Autodesk Inventor part; units mm, degrees
ref_plane "YZ Plane" through (0, 0, 0) normal (1, 0, 0) x (0, 1, 0)
ref_plane "XZ Plane" through (0, 0, 0) normal (0, 1, 0) x (-1, 0, 0)
ref_plane "XY Plane" through (0, 0, 0) normal (0, 0, 1) x (1, 0, 0)
sketch "Sketch1" plane through (0, 0, 0) normal (0, 0, 1) x (1, 0, 0)
  circle A0 centre (0, 0) radius 3.302
  line L0 (0, 0) -> (0, 9.525)
  circle A1 centre (0, 9.525) radius 1.5875
  circle A2 centre (-8.2489, -4.7625) radius 1.5875
  circle A3 centre (8.2489, -4.7625) radius 1.5875
  circle A4 centre (0, 0) radius 12.7
  dimension "d0" = 6.604
  dimension "d1" = 9.525
  dimension "d2" = 3.175
  dimension "d5" = 360
  dimension "d7" = 25.4
extrude "Extrusion1" add sketch "Sketch1" along normal blind 3.175
sketch "Sketch2" plane through (0, 0, 3.175) normal (0, 0, 1) x (1, 0, 0)
  circle A0 centre (0, 0) radius 3.302
  circle A1 centre (8.2489, -4.7625) radius 1.5875
  circle A2 centre (-8.2489, -4.7625) radius 1.5875
  circle A3 centre (0, 9.525) radius 1.5875
  circle A4 centre (0, 0) radius 12.7
  circle A5 centre (0, 0) radius 2.3813
  dimension "d10" = 4.7625
extrude "Extrusion2" add sketch "Sketch2" along normal blind 0.635 contours A0 | A4
chamfer "Chamfer1" distance 1.27 angle 45 3 edges at (-1.5875, 9.525, 0) (-9.8364, -4.7625, 0) (6.6614, -4.7625, 0)
sketch "Sketch3" plane through (0, 0, 0) normal (0, 0, -1) x (-1, 0, 0)
  line L0 (0, 0) -> (17.5976, 10.16)
  line L1 (0, 0) -> (20.32, 0) construction
  circle A0 centre (17.5976, 10.16) radius 11.1125
  circle A1 centre (-17.5976, 10.16) radius 11.1125
  circle A2 centre (0, -20.32) radius 11.1125
  dimension "d16" = 20.32
  dimension "d17" = 30
  dimension "d18" = 22.225
  dimension "d21" = 360
extrude "Extrusion3" cut sketch "Sketch3" against normal blind 25.4
fillet "Fillet1" radius 3.175 6 edges at (-12.6986, 0.1857, 1.905) (-6.5101, 10.9045, 1.905) (12.6986, 0.1857, 1.905) (6.5101, 10.9045, 1.905) (6.1885, -11.0902, 1.905) (-6.1885, -11.0902, 1.905)
properties part number "spoolPinionBearingHolder" material "ABS Plastic"
Source: CAD feature listing. Evaluate the final solid. Frame: model axes, mm. A direction names the side the tool comes from. Round coordinates to 2 decimals unless told otherwise and drop trailing zeros. Order: outer loops, then holes, each group sorted by start corner. A loop starts at its lowest first (then second) coordinate and runs counter-clockwise, first axis right, second up. Notation, with made-up numbers: (27.5, 46.25) -> (54.5, 46.25) arc R25 ccw to (54.5, 59.25) -> close; hole circle Ø8 at (71, 66.25). An arc over 180 degrees is marked (long way). One line per item, written item: value. Start each with the question number.
Q1. Pin query (flat end, axial travel): pin 1 (2 mm diameter, centred on y = -8, z = 2.5, fed in from +X); pin 2 (10 mm diameter, centred on x = -5, y = 3.5, fed in from -Z); pin 3 (5 mm diameter, centred on x = -8.25, y = -4.76, fed in from -Z). Return the tip coordinate at first contact, or that it passes through.
Q2. Access query for faces 5 (the cylindrical face through (3.05, 1.26, 1.57)), 6 (the flat face through (3, -1, 3.81)). Directions: +Z, -Z, +X, -X, +Y, -Y. A direction counts if a zero-diameter tool reaches every point of the face in a straight line with its end or side. Return the directions, or none.
Q3. Draft query along X for faces 1 (the cylindrical face through (-0.1, 12.7, 1.9)), 2 (the flat face through (0, -4, 0)), 3 (the cylindrical face through (-9.419, -5.835, 2.522)), 4 (the cylindrical face through (1.1, 2.11, 3.49)). Return one class per face: pulls with the +X half, pulls with the -X half, needs draft (parallel to the pull), parting line crosses it, or undercut.
Q4. Section query A-A (x = 0). Give the number of separate pieces and of enclosed holes in the cut face, plus the area to 3 significant figures.
Q5. Section query D-D (y = 5.75). Return the cut outline in (x, z), plus the area to 3 significant figures.
Q6. Material intervals for probe 1 along Y at (x, z) = (0, 1.3); probe 2 along Y at (x, z) = (0, 3.65); probe 3 along X at (y, z) = (-2.75, 0.55), sorted ascending.
Findings below:
1. pin 1: x = 10.6
1. pin 2: z = 0
1. pin 3: z = 0.35
2. face 5: -Z
2. face 6: +Z, +X, -X, +Y, -Y
3. face 1: parting line crosses it
3. face 2: needs draft
3. face 3: undercut
3. face 4: undercut
4. separate pieces: 3
4. enclosed holes: 0
4. area: 45.8 mm²
5. outline: (-7.4, 0) -> (7.4, 0) -> (7.4, 3.81) -> (-7.4, 3.81) -> close
5. area: 56.4 mm²
6. probe 1: -9.21 to -3.3, 3.3 to 7.94, 11.11 to 12.7
6. probe 2: -9.21 to -2.38, 2.38 to 7.94, 11.11 to 12.7
6. probe 3: -12.4 to -9.38, -7.12 to -1.83, 1.83 to 7.12, 9.38 to 12.4
